The listing builds one solid part. Answer for the finished solid, in the listing's coordinates (mm). A direction names the side the tool comes from. Give positions to 0.01 mm unless a question says otherwise; leave off trailing zeros. Write each loop counter-clockwise with the first axis right and the second up, starting at its lowest first coordinate (ties: lowest second). Pieces come first, ordered by that corner, then holes. Notation, with made-up numbers: (-32.5, 24) -> (4.5, 24) arc R26 cw to (4.5, 51) -> close; hole circle Ø10 at (13.25, 85.5). An arc over 180 degrees is marked (long way). One line per question, with ' | ' between items.
from build123d import *

# Parameters (mm, degrees)
BOSS_EXTRUDE1_DEPTH                  = 7
FILLET1_R                            = 8.5
FILLET2_R                            = 5.5
FILLET3_R                            = 13.5
SKETCH3_W                            = 27
SKETCH3_H                            = 13.5
CUT_EXTRUDE1_DEPTH                   = 1.8
CUT_EXTRUDE5_REACH                   = 37.882
SKETCH12_W                           = 12
SKETCH12_H                           = 13.5
CUT_EXTRUDE6_REACH                   = 37.882
SKETCH13_R                           = 1.1
SKETCH17_R                           = 2.1
CUT_EXTRUDE14_DEPTH                  = 4
FILLET4_R                            = 3
SHELL2_START                         = 3
SHELL2_DEPTH                         = 4
SHELL2_START_2                       = 4.8
SHELL2_2_DEPTH                       = 2.2
SKETCH18_W                           = 22
SKETCH18_H                           = 22
BOSS_EXTRUDE2_DEPTH                  = 9
SKETCH19_W                           = 18
SKETCH19_H                           = 18
CUT_EXTRUDE15_DEPTH                  = 9
SKETCH20_R                           = 5
CUT_EXTRUDE16_DEPTH                  = 3
FILLET5_R                            = 9
SKETCH21_R                           = 5
BOSS_EXTRUDE3_DEPTH                  = 2
CUT_EXTRUDE17_DEPTH                  = 1.5
CUT_EXTRUDE17_DIRECTION_2_REACH      = 40.659
CUT_EXTRUDE17_DIRECTION_2_END_RADIUS = 5
CUT_EXTRUDE18_REACH                  = 43.358
SKETCH23_R                           = 2.5


# Read off the part's stored shape, not the designer's step: Shell2
# Some blends are built 0.0001 mm under size
with BuildPart() as part:
    # Sketch2 → Boss-Extrude1 (new body)
    with BuildSketch(Plane(origin=(0, 0, 0), x_dir=(0, 0, -1), z_dir=(1, 0, 0))):
        Polygon((-13.5, -17.5), (13.5, -17.5), (13.5, 17.5), (5.5, 32.5), (-5.5, 32.5), (-13.5, 17.5), align=None)
    extrude(amount=BOSS_EXTRUDE1_DEPTH)

    # Fillet1
    fillet1_edges = [part.edges().sort_by_distance(p)[0] for p in [
        (3.5, 32.5, 5.5),
        (3.5, 32.5, -5.5),
    ]]
    fillet(fillet1_edges, radius=FILLET1_R)

    # Fillet2
    fillet2_edges = [part.edges().sort_by_distance(p)[0] for p in [
        (3.5, 17.5, -13.5),
        (3.5, 17.5, 13.5),
    ]]
    fillet(fillet2_edges, radius=FILLET2_R)

    # Fillet3
    fillet3_edges = [part.edges().sort_by_distance(p)[0] for p in [
        (3.5, -17.5, 13.5),
        (3.5, -17.5, -13.5),
    ]]
    fillet(fillet3_edges, radius=FILLET3_R - 0.0001)  # a hair under: the kernel refuses the full size

    # Sketch3 → Cut-Extrude1 (cut)
    with BuildSketch(Plane.ZY):
        with Locations((0, -10.75)):
            Rectangle(SKETCH3_W, SKETCH3_H)
    extrude(amount=-CUT_EXTRUDE1_DEPTH, mode=Mode.SUBTRACT)

    # Sketch12 → Cut-Extrude5 (cut, up to next)
    with BuildSketch(Plane(origin=(7, 0, 0), x_dir=(0, 0, -1), z_dir=(1, 0, 0)), mode=Mode.PRIVATE) as cut_extrude5_sk1:
        with Locations((0, -10.75)):
            Rectangle(SKETCH12_W, SKETCH12_H)
    cut_extrude5_tool1 = extrude(cut_extrude5_sk1.sketch, amount=-CUT_EXTRUDE5_REACH, mode=Mode.PRIVATE) & part.part
    add(cut_extrude5_tool1.solids().sort_by_distance((7, -10.75, 0))[0], mode=Mode.SUBTRACT)

    # Sketch13 → Cut-Extrude6 (cut, up to next)
    with BuildSketch(Plane.ZY, mode=Mode.PRIVATE) as cut_extrude6_sk1:
        with Locations((-7.5, 23.5)):
            Circle(SKETCH13_R)
    cut_extrude6_tool1 = extrude(cut_extrude6_sk1.sketch, amount=-CUT_EXTRUDE6_REACH, mode=Mode.PRIVATE) & part.part
    # Sketch13 → Cut-Extrude6 (cut, up to next)
    with BuildSketch(Plane.ZY, mode=Mode.PRIVATE) as cut_extrude6_sk2:
        with Locations((-10, -8.5)):
            Circle(SKETCH13_R)
    cut_extrude6_tool2 = extrude(cut_extrude6_sk2.sketch, amount=-CUT_EXTRUDE6_REACH, mode=Mode.PRIVATE) & part.part
    # Sketch13 → Cut-Extrude6 (cut, up to next)
    with BuildSketch(Plane.ZY, mode=Mode.PRIVATE) as cut_extrude6_sk3:
        with Locations((10, -8.5)):
            Circle(SKETCH13_R)
    cut_extrude6_tool3 = extrude(cut_extrude6_sk3.sketch, amount=-CUT_EXTRUDE6_REACH, mode=Mode.PRIVATE) & part.part
    # Sketch13 → Cut-Extrude6 (cut, up to next)
    with BuildSketch(Plane.ZY, mode=Mode.PRIVATE) as cut_extrude6_sk4:
        with Locations((7.5, 23.5)):
            Circle(SKETCH13_R)
    cut_extrude6_tool4 = extrude(cut_extrude6_sk4.sketch, amount=-CUT_EXTRUDE6_REACH, mode=Mode.PRIVATE) & part.part
    add(cut_extrude6_tool1.solids().sort_by_distance((0, 23.5, -7.5))[0], mode=Mode.SUBTRACT)
    add(cut_extrude6_tool2.solids().sort_by_distance((0, -8.5, -10))[0], mode=Mode.SUBTRACT)
    add(cut_extrude6_tool3.solids().sort_by_distance((0, -8.5, 10))[0], mode=Mode.SUBTRACT)
    add(cut_extrude6_tool4.solids().sort_by_distance((0, 23.5, 7.5))[0], mode=Mode.SUBTRACT)

    # Sketch17 → Cut-Extrude14 (cut)
    with BuildSketch(Plane.ZY):
        with Locations((-7.5, 23.5)):
            Circle(SKETCH17_R)
        with Locations((7.5, 23.5)):
            Circle(SKETCH17_R)
        with Locations((-10, -8.5)):
            Circle(SKETCH17_R)
        with Locations((10, -8.5)):
            Circle(SKETCH17_R)
    extrude(amount=-CUT_EXTRUDE14_DEPTH, mode=Mode.SUBTRACT)

    # Fillet4
    fillet4_edges = [part.edges().sort_by_distance(p)[0] for p in [
        (4.4, -16.093424605, -6),
        (4.4, -16.093424605, 6),
    ]]
    fillet(fillet4_edges, radius=FILLET4_R)

    # Shell2 outline → Shell2 (cut)
    with BuildSketch(Plane.YZ.offset(SHELL2_START)):
        with BuildLine():
            Line((17.301470588, -10.205882353), (18.775176121, -9.419906069))
            ThreePointArc((18.775176121, -9.419906069), (21.033978224, -3.035838645), (27.640649185, -4.522580929))
            ThreePointArc((27.640649185, -4.522580929), (29.013659867, -2.661241858), (29.5, -0.4))
            Line((29.5, -0.4), (29.5, 0.4))
            ThreePointArc((29.5, 0.4), (29.013659867, 2.661241858), (27.640649185, 4.522580929))
            ThreePointArc((27.640649185, 4.522580929), (21.033978224, 3.035838645), (18.775176121, 9.419906069))
            Line((18.775176121, 9.419906069), (17.301470588, 10.205882353))
            ThreePointArc((17.301470588, 10.205882353), (16.731339062, 10.42535625), (16.125, 10.5))
            Line((16.125, 10.5), (-1, 10.5))
            Line((-1, 10.5), (-1, -10.5))
            Line((-1, -10.5), (16.125, -10.5))
            ThreePointArc((16.125, -10.5), (16.731339062, -10.42535625), (17.301470588, -10.205882353))
        make_face()
    extrude(amount=SHELL2_DEPTH, mode=Mode.SUBTRACT)

    # Shell2 2 outline → Shell2 2 (cut)
    with BuildSketch(Plane.YZ.offset(SHELL2_START_2)):
        with BuildLine():
            Line((-3.424568984, -10.5), (-1, -10.5))
            Line((-1, -10.5), (-1, -9))
            Line((-1, -9), (-3.4990001, -9))
            ThreePointArc((-3.4990001, -9), (-3.406267086, -9.747245183), (-3.424568984, -10.5))
        make_face()
        with BuildLine():
            Line((-3.4990001, 9), (-1, 9))
            Line((-1, 9), (-1, 10.5))
            Line((-1, 10.5), (-3.424568984, 10.5))
            ThreePointArc((-3.424568984, 10.5), (-3.406267086, 9.747245183), (-3.4990001, 9))
        make_face()
    extrude(amount=SHELL2_2_DEPTH, mode=Mode.SUBTRACT)

    # Sketch18 → Boss-Extrude2 (add)
    with BuildSketch(Plane.ZY):
        with Locations((0, 7)):
            Rectangle(SKETCH18_W, SKETCH18_H)
    extrude(amount=BOSS_EXTRUDE2_DEPTH)

    # Sketch19 → Cut-Extrude15 (cut)
    with BuildSketch(Plane.ZY.offset(9)):
        with Locations((0, 7)):
            Rectangle(SKETCH19_W, SKETCH19_H)
    extrude(amount=-CUT_EXTRUDE15_DEPTH, mode=Mode.SUBTRACT)

    # Sketch20 → Cut-Extrude16 (cut)
    with BuildSketch(Plane.ZY):
        with Locations((0, 7)):
            Circle(SKETCH20_R)
    extrude(amount=-CUT_EXTRUDE16_DEPTH, mode=Mode.SUBTRACT)

    # Fillet5
    # the kernel refuses this fillet: 9 mm, written as the material it adds along each edge
    with BuildSketch(Plane(origin=(0, 16, -9), x_dir=(-1, 0, 0), z_dir=(0, -1, 0))) as fillet5_piece_1_section:
        with BuildLine():
            CenterArc((FILLET5_R, -FILLET5_R), FILLET5_R, 90, 90)
            Line((0, -FILLET5_R), (0, 0))
            Line((0, 0), (FILLET5_R, 0))
        make_face()
    fillet5_piece_1 = extrude(amount=18, mode=Mode.PRIVATE)
    fillet5_piece_1 = fillet5_piece_1 - Plane(origin=(-0.132604543, 7, 0), x_dir=(0, 0, 1), z_dir=(-1, 0, 0)) * Cylinder(5, 72, mode=Mode.PRIVATE)
    add(fillet5_piece_1)
    with BuildSketch(Plane(origin=(0, -2, 9), x_dir=(-1, 0, 0), z_dir=(0, 1, 0))) as fillet5_piece_2_section:
        with BuildLine():
            CenterArc((FILLET5_R, -FILLET5_R), FILLET5_R, 90, 90)
            Line((0, -FILLET5_R), (0, 0))
            Line((0, 0), (FILLET5_R, 0))
        make_face()
    fillet5_piece_2 = extrude(amount=18, mode=Mode.PRIVATE)
    fillet5_piece_2 = fillet5_piece_2 - Plane(origin=(-2.089358555, 7, 0), x_dir=(0, 0, 1), z_dir=(-1, 0, 0)) * Cylinder(5, 72, mode=Mode.PRIVATE)
    add(fillet5_piece_2)

    # Sketch21 → Boss-Extrude3 (add)
    with BuildSketch(Plane(origin=(0, 18, 0), x_dir=(1, 0, 0), z_dir=(0, 1, 0))):
        with Locations((-9, 0)):
            Circle(SKETCH21_R)
    boss_extrude3 = extrude(amount=-BOSS_EXTRUDE3_DEPTH)

    # Mirror1: Boss-Extrude3 across plane
    add(boss_extrude3.mirror(Plane.ZX.offset(7)))

    # Sketch22 → Cut-Extrude17 (cut)
    with BuildSketch(Plane.ZY.offset(9)):
        Polygon((-5, 16), (-5, 18), (-11, 18), (-11, -4), (-5, -4), (-5, -2), (5, -2), (5, -4), (11, -4), (11, 18), (5, 18), (5, 16), align=None)
    extrude(amount=-CUT_EXTRUDE17_DEPTH, mode=Mode.SUBTRACT)

    # Cut-Extrude17 direction 2: up to this cylinder (the profile starts inside it)
    cut_extrude17_direction_2_end = Plane(origin=(-9, 7, 0), z_dir=(0, 1, 0)) * Cylinder(CUT_EXTRUDE17_DIRECTION_2_END_RADIUS, 92.318, mode=Mode.PRIVATE)
    # Sketch22 → Cut-Extrude17 direction 2 (cut, up to the surface)
    with BuildSketch(Plane.ZY.offset(9), mode=Mode.PRIVATE) as cut_extrude17_direction_2_sk1:
        Polygon((-5, 16), (-5, 18), (-11, 18), (-11, -4), (-5, -4), (-5, -2), (5, -2), (5, -4), (11, -4), (11, 18), (5, 18), (5, 16), align=None)
    cut_extrude17_direction_2_tool1 = extrude(cut_extrude17_direction_2_sk1.sketch, amount=CUT_EXTRUDE17_DIRECTION_2_REACH, mode=Mode.PRIVATE) & cut_extrude17_direction_2_end
    add(cut_extrude17_direction_2_tool1.solids().sort_by_distance((-9, 7, 0))[0], mode=Mode.SUBTRACT)

    # Cut-Extrude18: up to this face of the body (flat: up to its plane)
    cut_extrude18_end = Plane(part.part.faces().sort_by_distance((-5.378131987, 18, 0))[0])
    # Sketch23 → Cut-Extrude18 (cut, up to the picked face)
    with BuildSketch(Plane.XZ.offset(4), mode=Mode.PRIVATE) as cut_extrude18_sk1:
        with Locations(Location((-9, 0, 0), (0, 0, 270))):
            Circle(SKETCH23_R)
    cut_extrude18_tool1 = split(extrude(cut_extrude18_sk1.sketch, amount=-CUT_EXTRUDE18_REACH, mode=Mode.PRIVATE), bisect_by=cut_extrude18_end, keep=Keep.BOTH, mode=Mode.PRIVATE)
    add(cut_extrude18_tool1.solids().sort_by(Axis((-9, -4, 0), (0, 1, 0)))[0], mode=Mode.SUBTRACT)


solid = part.part
Item 1: Consider line 1 (Z direction, x = 1.55, y = 7); line 2 (Y direction, x = 6.2, z = 7.5); line 3 (Y direction, x = -4.25, z = 0). Determine where each line is inside the solid, lowest interval first. Write a range as [from, to].
Answers below:
line 1: [-13.5, -5], [5, 13.5] | line 2: [-12.01, -1], [18.4, 22.4], [24.6, 28.67] | line 3: [-4, -2], [16, 18]
Item 2: Find section C-C (y = 7). Write down the section's boundary in (x, z).
Answers below:
outline: (-7.5, -11) -> (0, -11) -> (0, -13.5) -> (7, -13.5) -> (7, -10.5) -> (3, -10.5) -> (3, -5) -> (-1.52, -5) arc R9 cw to (-7.5, -8.87) -> close; (-7.5, 8.87) arc R9 cw to (-1.52, 5) -> (3, 5) -> (3, 10.5) -> (7, 10.5) -> (7, 13.5) -> (0, 13.5) -> (0, 11) -> (-7.5, 11) -> close
Item 3: Determine the mould class of faces 1 (the face through (1.21, 8.86, 4.64)), 2 (the face through (-4, 7, 11)), 3 (the face through (3.549, 31.255, -4.828)), 4 (the face through (2.885, -7.081, 8.452)) for opening direction Z: pulls with the +Z half, pulls with the -Z half, needs draft (parallel to the pull), parting line crosses it, or undercut.
Answers below:
face 1: undercut | face 2: pulls with the +Z half | face 3: pulls with the -Z half | face 4: undercut
Item 4: Find section B-B (x = 2.5). Write down the section's boundary in (y, z) (3 decimals).
Answers below:
outline: (-10.954, -11.571) arc R13.5 ccw to (-4, -13.5) -> (16.125, -13.5) arc R5.5 ccw to (18.713, -12.853) -> (28, -7.9) arc R8.5 ccw to (32.5, -0.4) -> (32.5, 0.4) arc R8.5 ccw to (28, 7.9) -> (18.713, 12.853) arc R5.5 ccw to (16.125, 13.5) -> (-4, 13.5) arc R13.5 ccw to (-10.954, 11.571) arc R3 ccw to (-9.408, 6) -> (-4, 6) -> (-4, -6) -> (-9.408, -6) arc R3 ccw to start; hole circle Ø4.2 at (-8.5, -10); hole circle Ø4.2 at (-8.5, 10); hole circle Ø10 at (7, 0); hole circle Ø4.2 at (23.5, -7.5); hole circle Ø4.2 at (23.5, 7.5)
Item 5: Flat-ended cylindrical pins translate along their axes: pin 1 (2 mm diameter, centred on x = 0.5, z = 7.5, fed in from +Y); pin 2 (3 mm diameter, centred on y = 4.5, z = -3.5, fed in from -X); pin 3 (3.5 mm diameter, centred on y = -8, z = -9.5, fed in from -X); pin 4 (1.3 mm diameter, centred on y = 23.5, z = -7.5, fed in from -X). Find the tip coordinate at first contact, or state that the pin passes through.
Answers below:
pin 1: y = 29.92 | pin 2: x = -1.52 | pin 3: x = 1.8 | pin 4: through
Item 6: Find section D-D (z = -1). Write down the section's boundary in (x, y).
Answers below:
outline: (-13.9, -4) -> (-11.29, -4) -> (-11.29, -2) -> (-13.9, -2) -> close; (-13.9, 16) -> (-11.29, 16) -> (-11.29, 18) -> (-13.9, 18) -> close; (-6.71, -4) -> (7, -4) -> (7, -1) -> (3, -1) -> (3, 2.1) -> (-0.06, 2.1) -> (-0.06, -2) -> (-6.71, -2) -> close; (-6.71, 16) -> (-0.06, 16) -> (-0.06, 11.9) -> (3, 11.9) -> (3, 29.47) -> (7, 29.47) -> (7, 32.48) -> (0, 32.48) -> (0, 18) -> (-6.71, 18) -> close
Item 7: A tool of negligible diameter and unlimited length cuts with its end or side. For faces 5 (the face through (3.45, 23.29, -10.41)), 6 (the face through (1.8, -7, -8)), 7 (the face through (4.8, -2, -10)), 8 (the face through (1.972, 24.919, 5.952)), 9 (the face through (5.479, 22.426, -7.738)), from which of +Z, -Z, +X, -X, +Y, -Y can it reach the whole face along a straight path? Write none if from no direction.
Answers below:
face 5: -Z, +X, -X, +Y | face 6: +Z, -Z, -X, -Y | face 7: +X | face 8: -X | face 9: +X, -X
Item 8: Find section A-A (y = 23.5). Write down the section's boundary in (x, z).
Answers below:
outline: (0, -10.3) -> (7, -10.3) -> (7, -8.6) -> (4, -8.6) -> (4, -9.6) -> (0, -9.6) -> close; (0, -5.4) -> (4, -5.4) -> (4, -6.4) -> (7, -6.4) -> (7, -2.4) -> (3, -2.4) -> (3, 2.4) -> (7, 2.4) -> (7, 6.4) -> (4, 6.4) -> (4, 5.4) -> (0, 5.4) -> close; (0, 9.6) -> (4, 9.6) -> (4, 8.6) -> (7, 8.6) -> (7, 10.3) -> (0, 10.3) -> close
